Design review of the part built by this model. Coordinates are the model's own, in mm. A direction names the side the tool comes from. Round coordinates to 2 decimals unless told otherwise and drop trailing zeros. Order: outer loops, then holes, each group sorted by start corner. A loop starts at its lowest first (then second) coordinate and runs counter-clockwise, first axis right, second up.
from build123d import *

# Parameters (mm, degrees)
MAINBODYS_W                           = 6.4
MAINBODYS_H                           = 0.8
MAIN_BODY_DEPTH                       = 14
BOTTOM_OF_MAIN_BODY_REACH             = 16.367
BOTTOM_OF_MAIN_BODY_DIRECTION_2_REACH = 16.367
TOPHOLES_R                            = 0.9
TOP_HOLE_DEPTH                        = 15.727185746
F_45_DEGREE_FLANGE_DEPTH              = 2
BOTTOM_FLAT_FLANGE_DEPTH              = 2
EXTENDEDBOTTOMFLANGES_W               = 3
EXTENDEDBOTTOMFLANGES_H               = 0.8
EXTENDED_BOTTOM_FLANGE_DEPTH          = 0.8
BOSSEDCYLINDERBODYS_R                 = 1.45
BOSSED_CYLINDER_BODY_DEPTH            = 0.8
C_MAIN_BODY_SIZE                      = 1


# Sheet-metal steps are written as plain solids
with BuildPart() as part:
    # MainBodyS → MAIN BODY (new body)
    with BuildSketch(Plane(origin=(0, 0, 0), x_dir=(1, 0, 0), z_dir=(0, 1, 0))):
        Rectangle(MAINBODYS_W, MAINBODYS_H)
    extrude(amount=MAIN_BODY_DEPTH)

    # BOTTOM OF MAIN BODY: up to this face of the body (flat: up to its plane)
    bottom_of_main_body_end = Plane(part.part.faces().sort_by_distance((0, 7, 0.4))[0])
    # BottomMainBodyS → BOTTOM OF MAIN BODY (add, up to the picked face)
    with BuildSketch(Plane.XY, mode=Mode.PRIVATE) as bottom_of_main_body_sk1:
        Polygon((0, 0), (4, 0), (4, -2), (4.5, -5), (2.9, -5), (1.5, -2.2), (0, -2.2), align=None)
    bottom_of_main_body_tool1 = split(extrude(bottom_of_main_body_sk1.sketch, amount=BOTTOM_OF_MAIN_BODY_REACH, mode=Mode.PRIVATE), bisect_by=bottom_of_main_body_end, keep=Keep.BOTH, mode=Mode.PRIVATE)
    bottom_of_main_body = bottom_of_main_body_tool1.solids().sort_by(Axis((2.475691, -2.049989, 0), (0, 0, 1)))[0]
    add(bottom_of_main_body)

    # BOTTOM OF MAIN BODY direction 2: up to this face of the body (flat: up to its plane)
    bottom_of_main_body_direction_2_end = Plane(part.part.faces().sort_by_distance((0, 7, -0.4))[0])
    # BottomMainBodyS → BOTTOM OF MAIN BODY direction 2 (add, up to the picked face)
    with BuildSketch(Plane.XY, mode=Mode.PRIVATE) as bottom_of_main_body_direction_2_sk1:
        Polygon((0, 0), (4, 0), (4, -2), (4.5, -5), (2.9, -5), (1.5, -2.2), (0, -2.2), align=None)
    bottom_of_main_body_direction_2_tool1 = split(extrude(bottom_of_main_body_direction_2_sk1.sketch, amount=-BOTTOM_OF_MAIN_BODY_DIRECTION_2_REACH, mode=Mode.PRIVATE), bisect_by=bottom_of_main_body_direction_2_end, keep=Keep.BOTH, mode=Mode.PRIVATE)
    bottom_of_main_body_direction_2 = bottom_of_main_body_direction_2_tool1.solids().sort_by(Axis((2.475691, -2.049989, 0), (0, 0, -1)))[0]
    add(bottom_of_main_body_direction_2)

    # BMB HM: BOTTOM OF MAIN BODY, BOTTOM OF MAIN BODY direction 2 across plane
    add(bottom_of_main_body.mirror(Plane(origin=(0, 0, 0), x_dir=(0, 0, 1), z_dir=(1, 0, 0))))
    add(bottom_of_main_body_direction_2.mirror(Plane(origin=(0, 0, 0), x_dir=(0, 0, 1), z_dir=(1, 0, 0))))

    # TopHoleS → TOP HOLE (cut, through all)
    with BuildSketch(Plane.XY.offset(0.4)):
        with Locations((0, 10)):
            Circle(TOPHOLES_R)
    extrude(amount=-TOP_HOLE_DEPTH, mode=Mode.SUBTRACT)

    # 45 DEGREE FLANGE section (across the edge) → 45 DEGREE FLANGE (add)
    with BuildSketch(Plane(origin=(1, -2.365685425, -0.4), x_dir=(0, 0.7071067811865438, -0.7071067811865512), z_dir=(-1, 0, 0))):
        with BuildLine():
            Line((-0.8, 0.165685425), (-0.8, 2.2))
            Line((-0.8, 2.2), (0, 2.2))
            Line((0, 2.2), (0, 0.165685425))
            ThreePointArc((0, 0.165685425), (0.030448187, 0.012612052), (0.117157288, -0.117157288))
            Line((0.117157288, -0.117157288), (-0.448528137, -0.682842712))
            ThreePointArc((-0.448528137, -0.682842712), (-0.708655439, -0.293534694), (-0.8, 0.165685425))
        make_face()
    extrude(amount=F_45_DEGREE_FLANGE_DEPTH)

    # BOTTOM FLAT FLANGE section (across the edge) → BOTTOM FLAT FLANGE (add)
    with BuildSketch(Plane(origin=(-1, -5.169848481, -2.072792206), x_dir=(0, 1, 0), z_dir=(1, 0, 0))):
        with BuildLine():
            Line((-0.8, 0.965685425), (-0.8, 1.5))
            Line((-0.8, 1.5), (0, 1.5))
            Line((0, 1.5), (0, 0.965685425))
            ThreePointArc((0, 0.965685425), (0.246926627, 0.596133612), (0.682842712, 0.682842712))
            Line((0.682842712, 0.682842712), (1.248528137, 0.117157288))
            ThreePointArc((1.248528137, 0.117157288), (-0.059220119, -0.142970014), (-0.8, 0.965685425))
        make_face()
    extrude(amount=BOTTOM_FLAT_FLANGE_DEPTH)

    # ExtendedBottomFlangeS → EXTENDED BOTTOM FLANGE (add)
    with BuildSketch(Plane.XY.offset(-0.572792206)):
        with Locations((0, -5.569848481)):
            Rectangle(EXTENDEDBOTTOMFLANGES_W, EXTENDEDBOTTOMFLANGES_H)
    extrude(amount=EXTENDED_BOTTOM_FLANGE_DEPTH)

    # BossedCylinderBodyS → BOSSED  CYLINDER BODY (add)
    with BuildSketch(Plane.XZ.offset(5.969848481)):
        with BuildLine():
            Line((-1.5, 0.227207794), (1.5, 0.227207794))
            ThreePointArc((1.5, 0.227207794), (0, 4.614344857), (-1.5, 0.227207794))
        make_face()
        with Locations(Location((0, 2.164344857, 0), (0, 0, 270))):
            Circle(BOSSEDCYLINDERBODYS_R, mode=Mode.SUBTRACT)
    extrude(amount=-BOSSED_CYLINDER_BODY_DEPTH)

    # C MAIN BODY
    c_main_body_edges = [part.edges().sort_by_distance(p)[0] for p in [
        (-3.2, 14, 0),
        (3.2, 14, 0),
    ]]
    chamfer(c_main_body_edges, length=C_MAIN_BODY_SIZE)


solid = part.part
1) Take a section at B-B on y = 10. Give the boundary of the cut face in (x, z), plus the area to 3 significant figures.
Results:
outline: (-3.2, -0.4) - (-0.9, -0.4) - (-0.9, 0.4) - (-3.2, 0.4) - close; (0.9, -0.4) - (3.2, -0.4) - (3.2, 0.4) - (0.9, 0.4) - close
area: 3.68 mm2
2) Take a section at A-A on x = 0. Give the boundary of the cut face in (y, z).
Results:
outline: (-5.97, -1.11) arc R1.2 ccw to (-3.92, -1.96) - (-2.48, -0.52) arc R0.4 cw to (-2.2, -0.4) - (9.1, -0.4) - (9.1, 0.4) - (-2.2, 0.4) arc R1.2 ccw to (-3.05, 0.05) - (-4.49, -1.39) arc R0.4 cw to (-5.17, -1.11) - (-5.17, 0.71) - (-5.97, 0.71) - close; (-5.97, 3.61) - (-5.17, 3.61) - (-5.17, 4.61) - (-5.97, 4.61) - close; (10.9, -0.4) - (14, -0.4) - (14, 0.4) - (10.9, 0.4) - close
3) To check wall thickness, follow line 1 along Y through (x, z) = (0, 0.05); line 2 along Y through (x, z) = (0, 0.2); line 3 along Z through (x, y) = (-2.25, 7.25). State the ranges of each line that lie inside material, in increasing order.
Results:
line 1: y = -5.97 to -5.17, -3.05 to 9.1, 10.9 to 14
line 2: y = -5.97 to -5.17, -2.86 to 9.1, 10.9 to 14
line 3: z = -0.4 to 0.4
4) The part is to be moulded in two halves that separate along X. For faces 4 (the face through (0.014, -3.758, -0.661)), 5 (the face through (-0.014, -5.211, -2.223)), 6 (the face through (-2.7, 13.5, 0)), say which applies: released by +X, released by -X, zero draft, split by the parting line, or undercut.
Results:
face 4: undercut
face 5: zero draft
face 6: released by -X
5) Clearance check with flat-ended pins moving along their axes: P1, Ø2, axis at x = -3, y = -2, coming from the -Z side; P2, Ø3, axis at y = -4, z = -0.5, coming from the -X side; P3, Ø1, axis at x = -2, z = 1, coming from the +Y side; P4, Ø0.6, axis at y = -5.5, z = 0, coming from the -X side. State where each tip first meets the part, or that it passes through.
Results:
P1: stops at z = -0.4
P2: stops at x = -4.5
P3: stops at y = -5.17
P4: stops at x = -1.59
6) Take a section at C-C on z = 2.5. Give the boundary of the cut face in (x, y), plus the area to 3 significant figures.
Results:
outline: (-2.43, -5.97) - (-1.41, -5.97) - (-1.41, -5.17) - (-2.43, -5.17) - close; (1.41, -5.97) - (2.43, -5.97) - (2.43, -5.17) - (1.41, -5.17) - close
area: 1.63 mm2
7) For faces 1 (the face through (0, 5, 0.4)), 2 (the face through (-1, -4.06, -1.24)), 3 (the face through (0.014, -2.653, 0.311)), list the 3-axis set-ups (+Z, -Z, +X, -X, +Y, -Y) from which the entire face can be reached by the end or side of a thin tool; tool diameter is ignored.
Results:
face 1: +Z, +X, -X, +Y
face 2: -Z
face 3: +Z
8) Take a section at D-D on x = 3.5. Give the boundary of the cut face in (y, z).
Results:
outline: (-5, -0.4) - (0, -0.4) - (0, 0.4) - (-5, 0.4) - close
